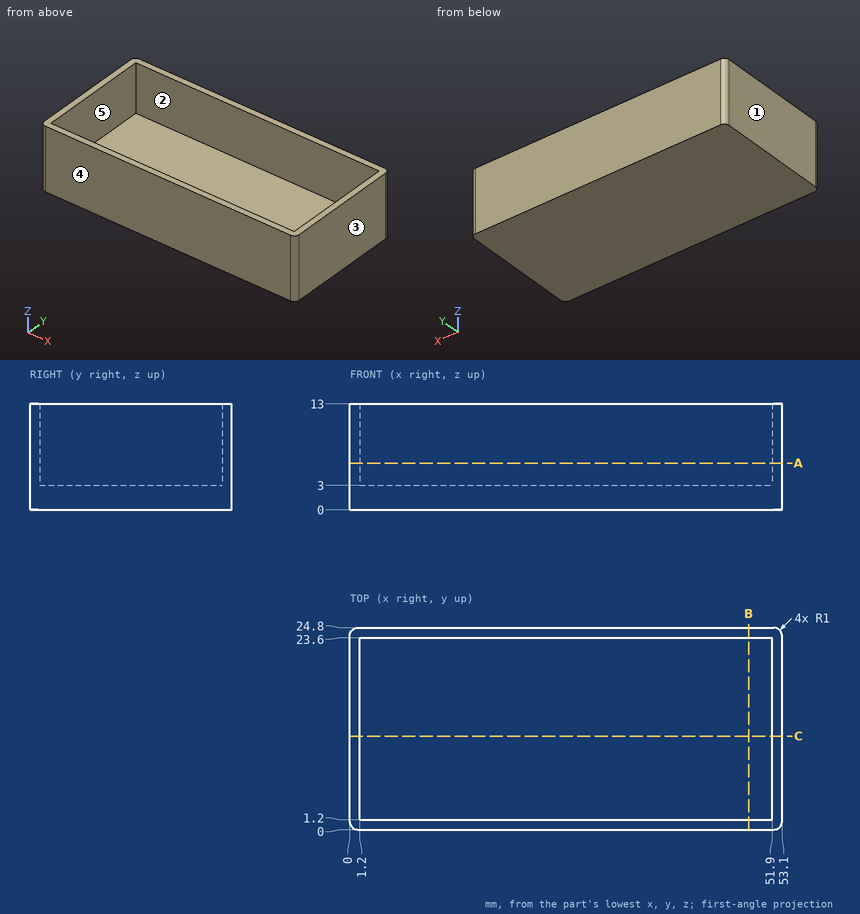
For this review, use the dimensioned drawing (mm, ordinates from the lowest corner) and the shaded views. A direction names the side the tool comes from. Give positions to 0.01 mm unless a question says otherwise; leave off trailing zeros. Order: outer loops, then holes, each group sorted by start corner. A loop starts at its lowest first (then second) coordinate and runs counter-clockwise, first axis right, second up. Notation, with made-up numbers: (-20, 41) -> (33, 41) arc R27 cw to (33, 70) -> close; hole circle Ø10 at (19.25, 36). An arc over 180 degrees is marked (long way). Write item = value, one per line. Start each with the question number.
(1) Draft analysis for pull direction X (two halves, no side actions). For the marked faces 1, 2 and 3, state which applies: +X half, -X half, draft (parallel to the pull), parting line (faces both ways), or undercut.
(2) Tool access review of the marked faces 4 and 5: name each direction out of +Z, -Z, +X, -X, +Y, -Y from which nothing blocks a thin tool from reaching the whole face with its end or side.
(3) For L1, parallel to X at y = 10, z = 5.5; L2, parallel to Y at x = 24.5, z = 8.5; L3, parallel to Z at x = 42.5, y = 16, list the stretches that pass through material, from the lowest coordinate up. Write a range as from..to.
(4) For pin 1 Ø1 at (x, y) = (20, 18.5) entering from +Z; pin 2 Ø8 at (x, y) = (18.5, 17.5) entering from -Z, all flat-tipped, find the tip position at first contact; note any pin that passes through.
(5) Take a section at A-A (z = 5.75). Write out the cut boundary in (x, y), plus the area to 3 significant figures.
(6) Take a section at C-C (y = 11.5). Write out the cut boundary in (x, z), plus the area to 3 significant figures.
(7) Take a section at B-B (x = 49). Write out the cut boundary in (y, z).
Returned:
q1.face_1 = -X half
q1.face_2 = undercut
q1.face_3 = +X half
q2.face_4 = +Z, -Z, +X, -X, -Y
q2.face_5 = +Z
q3.L1 = 0..1.2, 51.9..53.1
q3.L2 = 0..1.2, 23.6..24.8
q3.L3 = 0..3
q4.pin_1 = 3
q4.pin_2 = 0
q5.outline = (0, 1) arc R1 ccw to (1, 0) -> (52.1, 0) arc R1 ccw to (53.1, 1) -> (53.1, 23.8) arc R1 ccw to (52.1, 24.8) -> (1, 24.8) arc R1 ccw to (0, 23.8) -> close; hole (1.2, 1.2) -> (51.9, 1.2) -> (51.9, 23.6) -> (1.2, 23.6) -> close
q5.area = 180 mm²
q6.outline = (0, 0) -> (53.1, 0) -> (53.1, 13) -> (51.9, 13) -> (51.9, 3) -> (1.2, 3) -> (1.2, 13) -> (0, 13) -> close
q6.area = 183 mm²
q7.outline = (0, 0) -> (24.8, 0) -> (24.8, 13) -> (23.6, 13) -> (23.6, 3) -> (1.2, 3) -> (1.2, 13) -> (0, 13) -> close
